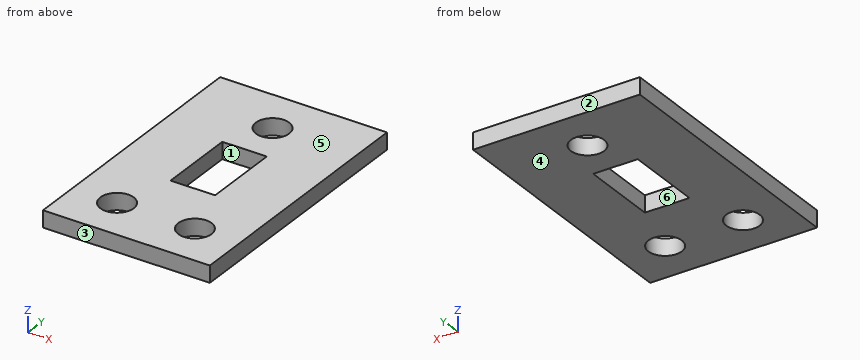
```python
from build123d import *

# Parameters (mm, degrees)
ESQUISSE1_W      = 15
ESQUISSE1_H      = 24
EXTRUSION1_DEPTH = 1.5
ESQUISSE2_R      = 1.5
ESQUISSE2_W      = 4
ESQUISSE2_H      = 7
EXTRUSION2_DEPTH = 2


with BuildPart() as part:
    # Esquisse1 → Extrusion1 (new body)
    with BuildSketch(Plane.XY):
        with Locations((-5.045528485, 20.953157895)):
            Rectangle(ESQUISSE1_W, ESQUISSE1_H)
    extrude(amount=EXTRUSION1_DEPTH)

    # Esquisse2 → Extrusion2 (cut)
    with BuildSketch(Plane.XY.offset(1.5)):
        with Locations((-8.545528485, 12.953157895)):
            Circle(ESQUISSE2_R)
        with Locations((-1.545528485, 12.953157895)):
            Circle(ESQUISSE2_R)
        with Locations((-5.045528485, 28.747386529)):
            Circle(ESQUISSE2_R)
        with Locations((-5.045528485, 21.453157895)):
            Rectangle(ESQUISSE2_W, ESQUISSE2_H)
    extrude(amount=-EXTRUSION2_DEPTH, mode=Mode.SUBTRACT)


solid = part.part
```
Verification items for the finished model (mm, model axes). Face numbers are marked on the shaded views. A direction names the side the tool comes from. Round coordinates to 2 decimals unless told otherwise and drop trailing zeros. Write each loop counter-clockwise with the first axis right and the second up, starting at its lowest first coordinate (ties: lowest second). Pieces come first, ordered by that corner, then holes.
1. Section check D-D on z = 1.15. Enter the section's corners in (x, y), plus the area to 3 significant figures.
2. Section check C-C on y = 12.25. Enter the section's corners in (x, z), plus the area to 3 significant figures.
3. Section check B-B on x = -4.75. Enter the section's corners in (y, z).
4. Access from +Z, -Z, +X, -X, +Y, -Y to the whole of each face (thin tool, end or side, straight path). Record for the marked faces 5 and 6.
5. Section check A-A on y = 19.25. Enter the section's corners in (x, z).
6. Scan lines: L1, parallel to X at y = 21.75, z = 0.5; L2, parallel to Y at x = -4.25, z = 1.3; L3, parallel to X at y = 27.5, z = 0.75. Record each from-to range of solid material in increasing order.
7. Draft check along Y on the marked faces 1, 2, 3 and 4. Enter one of: +Y half, -Y half, draft (parallel to the pull), parting line (faces both ways), or undercut.
Answer:
1. outline: (-12.55, 8.95) - (2.45, 8.95) - (2.45, 32.95) - (-12.55, 32.95) - close; hole circle Ø3 at (-8.55, 12.95); hole (-7.05, 17.95) - (-3.05, 17.95) - (-3.05, 24.95) - (-7.05, 24.95) - close; hole circle Ø3 at (-5.05, 28.75); hole circle Ø3 at (-1.55, 12.95)
1. area: 311 mm2
2. outline: (-12.55, 0) - (-9.87, 0) - (-9.87, 1.5) - (-12.55, 1.5) - close; (-7.22, 0) - (-2.87, 0) - (-2.87, 1.5) - (-7.22, 1.5) - close; (-0.22, 0) - (2.45, 0) - (2.45, 1.5) - (-0.22, 1.5) - close
2. area: 14.6 mm2
3. outline: (8.95, 0) - (17.95, 0) - (17.95, 1.5) - (8.95, 1.5) - close; (24.95, 0) - (27.28, 0) - (27.28, 1.5) - (24.95, 1.5) - close; (30.22, 0) - (32.95, 0) - (32.95, 1.5) - (30.22, 1.5) - close
4. face 5: +Z, +X, -X, +Y, -Y
4. face 6: +Z, -Z
5. outline: (-12.55, 0) - (-7.05, 0) - (-7.05, 1.5) - (-12.55, 1.5) - close; (-3.05, 0) - (2.45, 0) - (2.45, 1.5) - (-3.05, 1.5) - close
6. L1: x = -12.55 to -7.05, -3.05 to 2.45
6. L2: y = 8.95 to 17.95, 24.95 to 27.48, 30.02 to 32.95
6. L3: x = -12.55 to -5.88, -4.21 to 2.45
7. face 1: undercut
7. face 2: +Y half
7. face 3: -Y half
7. face 4: draft
